Study the drawing (mm; zero at the part's minimum x, y, z) and answer. Coordinates: 2 decimals unless noted, no trailing zeros. Loops run counter-clockwise (first coordinate to the right, second up) from the corner with the lowest first, then second, coordinate; pieces in that order, holes last. Notation, with made-up numbers: M 6.5,68 L 49.5,68 A10 ccw 49.5,79 Z; hole C -30.5,2 d2. An arc over 180 degrees is marked long. Use one line per item in the form item = value. Start each with the question number.
1. The part is cut by section A-A (z = 17). Give the number of separate pieces and of enclosed holes in the cut face, plus the area to 4 significant figures.
2. Flat-ended cylindrical pins translate along their axes: pin 1 (8 mm diameter, centred on x = 26, z = 23.5, fed in from -Y); pin 2 (3 mm diameter, centred on x = 54.1, z = 17, fed in from -Y); pin 3 (1.5 mm diameter, centred on y = 0.5, z = 30, fed in from +X). Find the tip coordinate at first contact, or state that the pin passes through.
3. The part is cut by section C-C (y = 0.6). Give the vertices of the cut face in (x, z), plus the area to 3 significant figures.
4. The part is cut by section D-D (z = 4). Give the vertices of the cut face in (x, y), plus the area to 3 significant figures.
5. Find the intervals of material crossed by probe 1 along X at (y, z) = (2.9, 19.5); probe 2 along X at (y, z) = (1.6, 17); probe 3 along Z at (x, y) = (51, 0.7), in increasing order. Write a range as [from, to].
6. The part is cut by section B-B (x = 46). Give the vertices of the cut face in (y, z), plus the area to 3 significant figures.
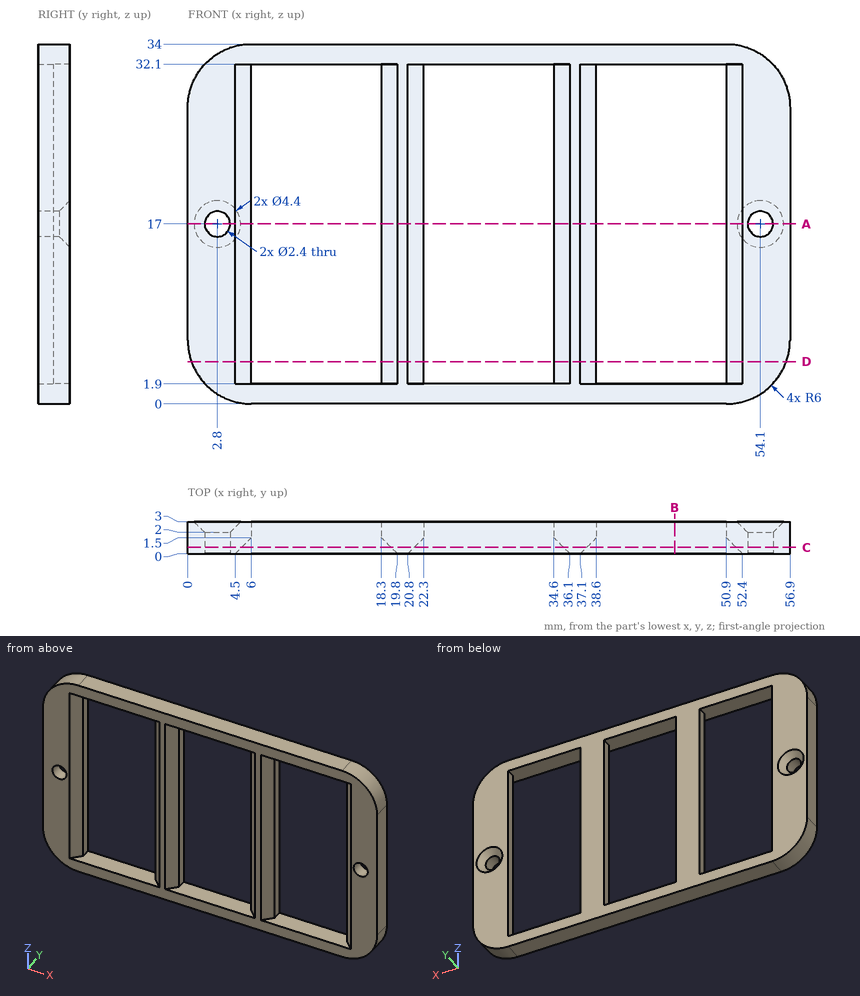
Computed values:
q1.separate_pieces = 6
q1.enclosed_holes = 0
q1.area = 36.85 mm²
q2.pin_1 = 1.2
q2.pin_2 = 0
q2.pin_3 = 56.77
q3.outline = M 0,6 A6 ccw 6,0 L 50.9,0 A6 ccw 56.9,6 L 56.9,28 A6 ccw 50.9,34 L 6,34 A6 ccw 0,28 Z; hole C 2.8,17 d2.4; hole M 5.1,1.9 L 19.2,1.9 L 19.2,32.1 L 5.1,32.1 Z; hole M 21.4,1.9 L 35.5,1.9 L 35.5,32.1 L 21.4,32.1 Z; hole M 37.7,1.9 L 51.8,1.9 L 51.8,32.1 L 37.7,32.1 Z; hole C 54.1,17 d2.4
q3.area = 617 mm²
q4.outline = M 0.34,0 L 4.5,0 L 6,1.5 L 6,3 L 0.34,3 Z; M 18.3,1.5 L 19.8,0 L 20.8,0 L 22.3,1.5 L 22.3,3 L 18.3,3 Z; M 34.6,1.5 L 36.1,0 L 37.1,0 L 38.6,1.5 L 38.6,3 L 34.6,3 Z; M 50.9,1.5 L 52.4,0 L 56.56,0 L 56.56,3 L 50.9,3 Z
q4.area = 51.2 mm²
q5.probe_1 = [0, 6], [18.3, 22.3], [34.6, 38.6], [50.9, 56.9]
q5.probe_2 = [0, 1.6], [4, 6], [18.3, 22.3], [34.6, 38.6], [50.9, 52.9], [55.3, 56.9]
q5.probe_3 = [0, 1.9], [32.1, 34]
q6.outline = M 0,0 L 3,0 L 3,1.9 L 0,1.9 Z; M 0,32.1 L 3,32.1 L 3,34 L 0,34 Z
q6.area = 11.4 mm²
